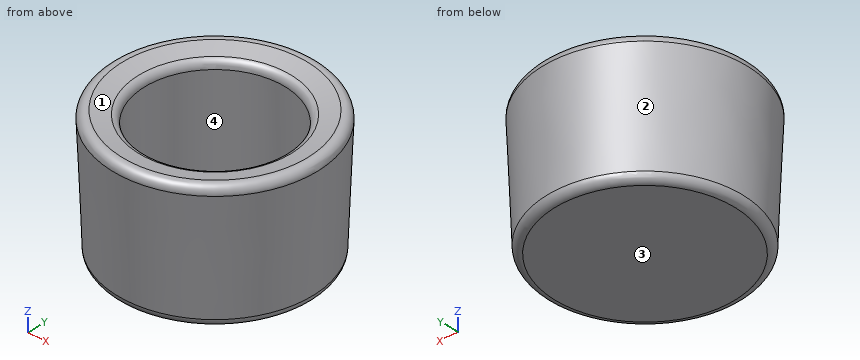
```python
from build123d import *


with BuildPart() as f1:
    # F0 (on Right) → F1 (revolve)
    with BuildSketch(Plane.YZ):
        with BuildLine():
            ThreePointArc((-35.643776, 49.074506), (-38.247983, 48.47563), (-39.341498, 46.03744))
            Line((-39.341498, 46.03744), (-37.615204, 2.880096))
            ThreePointArc((-37.615204, 2.880096), (-36.696097, 0.836702), (-34.617601, 0))
            Line((-34.617601, 0), (0, 0))
            Line((0, 0), (0, 3))
            Line((0, 3), (-25, 3))
            ThreePointArc((-25, 3), (-26.414214, 3.585786), (-27, 5))
            Line((-27, 5), (-27, 44.63481))
            ThreePointArc((-27, 44.63481), (-27.644118, 46.492179), (-29.299881, 47.551971))
            Line((-29.299881, 47.551971), (-35.643776, 49.074506))
        make_face()
    revolve(axis=Axis((0, 0, 1.5), (0, 0, 1)))


solid = f1.part
```
Could you check a few things on this model? Use its own coordinates, in mm. Face numbers are marked on the shaded views. Round coordinates to 2 decimals unless told otherwise and drop trailing zeros. Loops run counter-clockwise (first coordinate to the right, second up) from the corner with the lowest first, then second, coordinate; pieces in that order, holes last. Notation, with made-up numbers: (-5.5, -25.5) - (48.5, -25.5) arc R20 ccw to (48.5, -16.5) - close; hole circle Ø11 at (89.5, 77.25). An arc over 180 degrees is marked (long way). Use CSV: the item, a comma, the result in double quotes.
Item 1: I need wall thicknesses on L1, parallel to Z at x = 23, y = 4; L2, parallel to X at y = 0, z = 34; L3, parallel to X at y = 1.5, z = 25.5. Which ranges of each line are inside material? Lowest first, please. Write a range as [from, to].
Here are the results:
L1,"z = [0, 3]"
L2,"x = [-38.86, -27], [27, 38.86]"
L3,"x = [-38.49, -26.96], [26.96, 38.49]"
Item 2: Will these pins go through, and if not, where does the flat tip stop? pin 1 (5 mm diameter, centred on x = -11, y = 14, fed in from +Z); pin 2 (6 mm diameter, centred on y = -28, z = 27, fed in from -X); pin 3 (2 mm diameter, centred on y = -30.5, z = 40.5, fed in from -X).
Here are the results:
pin 1,"stops at z = 3"
pin 2,"stops at x = -29.39"
pin 3,"stops at x = -25.69"
Item 3: If we section it at D-D on z = 43.5: List the corners of the cut face in (x, y) for me.
Here are the results:
outline,"circle Ø78.48 at (0, 0); hole circle Ø54 at (0, 0)"
Item 4: If we section it at B-B on z = 16: List the corners of the cut face in (x, y) for me, then the cut area to 3 significant figures.
Here are the results:
outline,"circle Ø76.28 at (0, 0); hole circle Ø54 at (0, 0)"
area,"2,280 mm²"
Item 5: If we mould it in two halves opening along Y, with no side actions, what happens to the marked faces 1, 2, 3 and 4? For each: pulls with the +Y half, pulls with the -Y half, needs draft (parallel to the pull), parting line crosses it, or undercut.
Here are the results:
face 1,"undercut"
face 2,"parting line crosses it"
face 3,"needs draft"
face 4,"undercut"
Item 6: If we section it at A-A on y = 0: List the corners of the cut face in (x, z) for me, then the cut area to 3 significant figures.
Here are the results:
outline,"(-39.34, 46.04) - (-37.62, 2.88) arc R3 ccw to (-34.62, 0) - (34.62, 0) arc R3 ccw to (37.62, 2.88) - (39.34, 46.04) arc R3 ccw to (35.64, 49.07) - (29.3, 47.55) arc R3 ccw to (27, 44.63) - (27, 5) arc R2 cw to (25, 3) - (-25, 3) arc R2 cw to (-27, 5) - (-27, 44.63) arc R3 ccw to (-29.3, 47.55) - (-35.64, 49.07) arc R3 ccw to start"
area,"1,260 mm²"
